```python
from build123d import *

# Parameters (mm, degrees)
F0_R          = 2.5
F1_DEPTH      = 3
F2_DEPTH      = 5
F2_DEPTH_BACK = 45
F3_DEPTH      = 40
F4_START      = -37
F4_DEPTH      = 3


with BuildPart() as f1:
    # F0 (on Front) → F1 (new body)
    with BuildSketch(Plane.XZ):
        Polygon((-13, 42.7573593129), (-16, 39.7573593129), (-16, 2), (-13, 2), align=None)
        with BuildLine():
            Line((13, 2), (13, 42.7573593129))
            Line((13, 42.7573593129), (0, 55.7573593129))
            Line((0, 55.7573593129), (-13, 42.7573593129))
            Line((-13, 42.7573593129), (-13, 2))
            Line((-13, 2), (-9, 2))
            Line((-9, 2), (-9, 31.7573593129))
            ThreePointArc((-9, 31.7573593129), (0, 40.7573593129), (9, 31.7573593129))
            Line((9, 31.7573593129), (9, 2))
            Line((9, 2), (13, 2))
        make_face()
        with Locations((0, 46.9705627485)):
            Circle(F0_R, mode=Mode.SUBTRACT)
        Polygon((16, 2), (16, 39.7573593129), (13, 42.7573593129), (13, 2), align=None)
    extrude(amount=-F1_DEPTH)

    # F0 (on Front) → F2 (join, two sides)
    with BuildSketch(Plane.XZ) as f2_sk:
        Polygon((25, 35), (0, 60), (-25, 35), (-22.8786796564, 32.8786796564), (-16, 39.7573593129), (-13, 42.7573593129), (0, 55.7573593129), (13, 42.7573593129), (16, 39.7573593129), (22.8786796564, 32.8786796564), align=None)
    extrude(amount=F2_DEPTH)
    extrude(f2_sk.sketch, amount=-F2_DEPTH_BACK)

    # F0 (on Front) → F3 (join)
    with BuildSketch(Plane.XZ):
        Polygon((-13, 42.7573593129), (-16, 39.7573593129), (-16, 2), (-13, 2), align=None)
        Polygon((16, 2), (16, 39.7573593129), (13, 42.7573593129), (13, 2), align=None)
    extrude(amount=-F3_DEPTH)

    # F0 (on Front) → F4 (join)
    with BuildSketch(Plane.XZ.offset(F4_START)):
        with BuildLine():
            Line((13, 2), (13, 42.7573593129))
            Line((13, 42.7573593129), (0, 55.7573593129))
            Line((0, 55.7573593129), (-13, 42.7573593129))
            Line((-13, 42.7573593129), (-13, 2))
            Line((-13, 2), (-9, 2))
            Line((-9, 2), (-9, 31.7573593129))
            ThreePointArc((-9, 31.7573593129), (0, 40.7573593129), (9, 31.7573593129))
            Line((9, 31.7573593129), (9, 2))
            Line((9, 2), (13, 2))
        make_face()
        with Locations((0, 46.9705627485)):
            Circle(F0_R, mode=Mode.SUBTRACT)
        with BuildLine():
            Line((-9, 2), (9, 2))
            Line((9, 2), (9, 31.7573593129))
            ThreePointArc((9, 31.7573593129), (0, 40.7573593129), (-9, 31.7573593129))
            Line((-9, 31.7573593129), (-9, 2))
        make_face()
    extrude(amount=-F4_DEPTH)


solid = f1.part
```
For this review, take the finished solid that the model builds, in its own axes (mm). A direction names the side the tool comes from. Round coordinates to 2 decimals unless told otherwise and drop trailing zeros. Write each loop counter-clockwise with the first axis right and the second up, starting at its lowest first coordinate (ties: lowest second). Pieces come first, ordered by that corner, then holes. Notation, with made-up numbers: (5.5, -27) - (61.5, -27) arc R8 ccw to (61.5, -14) - close; hole circle Ø8 at (50, 35.5). An arc over 180 degrees is marked (long way). Answer as a JSON object with one key per item and string values.
1. Draft analysis for pull direction Z (two halves, no side actions). For faces 1 (the face through (24, 20, 34)), 2 (the face through (-0.54, 38.48, 44.53)), 3 (the face through (13, 20, 47)), state which applies: +Z half, -Z half, draft (parallel to the pull), parting line (faces both ways), or undercut.
Response values:
{"face 1": "-Z half", "face 2": "undercut", "face 3": "+Z half"}
2. We need section A-A on z = 25. Give the boundary of the cut face in (x, y).
Response values:
{"outline": "(-16, 0) - (-9, 0) - (-9, 3) - (-13, 3) - (-13, 37) - (13, 37) - (13, 3) - (9, 3) - (9, 0) - (16, 0) - (16, 40) - (-16, 40) - close"}
3. Tool access review of faces 4 (the face through (-16, 20, 21)), 5 (the face through (-11, 0, 29)), 6 (the face through (0, 40, 23)), 7 (the face through (13, 20, 23)): name each direction out of +Z, -Z, +X, -X, +Y, -Y from which nothing blocks a thin tool from reaching the whole face with its end or side.
Response values:
{"face 4": "-Z, +Y, -Y", "face 5": "-Z, -Y", "face 6": "-Z, +Y", "face 7": "-Z"}
4. We need section C-C on x = 15. Give the boundary of the cut face in (y, z), then the cut area to 3 significant figures.
Response values:
{"outline": "(-5, 40.76) - (0, 40.76) - (0, 2) - (40, 2) - (40, 40.76) - (45, 40.76) - (45, 45) - (-5, 45) - close", "area": "1,760 mm2"}
5. We need section D-D on z = 36.5. Give the boundary of the cut face in (x, y).
Response values:
{"outline": "(-23.5, -5) - (-19.26, -5) - (-19.26, 45) - (-23.5, 45) - close; (-16, 0) - (-7.65, 0) - (-7.65, 3) - (-13, 3) - (-13, 37) - (13, 37) - (13, 3) - (7.65, 3) - (7.65, 0) - (16, 0) - (16, 40) - (-16, 40) - close; (19.26, -5) - (23.5, -5) - (23.5, 45) - (19.26, 45) - close"}
6. For pin 1 Ø5 at (x, y) = (9.5, 9) entering from +Z; pin 2 Ø8 at (x, z) = (0, 46.97) entering from +Y; pin 3 Ø3 at (x, z) = (-9.5, 27.5) entering from -Y; pin 4 Ø8 at (x, z) = (-16.5, 53.5) entering from -Y, all flat-tipped, find the tip position at first contact; note any pin that passes through.
Response values:
{"pin 1": "stops at z = 53", "pin 2": "stops at y = 40", "pin 3": "stops at y = 0", "pin 4": "passes through"}
7. We need section B-B on y = -1.5. Give the boundary of the cut face in (x, z).
Response values:
{"outline": "(-25, 35) - (-22.88, 32.88) - (0, 55.76) - (22.88, 32.88) - (25, 35) - (0, 60) - close"}
8. To check wall thickness, follow line 1 along X through (y, z) = (25.5, 32.5); line 2 along Z through (x, y) = (0, 39); line 3 along Z through (x, y) = (0, 2.15). State the ranges of each line that lie inside material, in increasing order.
Response values:
{"line 1": "x = -16 to -13, 13 to 16", "line 2": "z = 2 to 44.47, 49.47 to 60", "line 3": "z = 40.76 to 44.47, 49.47 to 60"}
